Part model, mm, in its own coordinate system. A direction names the side the tool comes from. Coordinates: 2 decimals unless noted, no trailing zeros. Order: outer loops, then holes, each group sorted by start corner. A loop starts at its lowest first (then second) coordinate and runs counter-clockwise, first axis right, second up.
from build123d import *

# Parameters (mm, degrees)
FILLET_1_R = 1


with BuildPart() as part:
    # Эскиз1 → Повернуть1 (revolve)
    with BuildSketch(Plane.XY):
        Polygon((2.5, 0), (2.5, -30), (4.5, -30), (4.5, -0.828427125), (25.328427125, 20), (22.5, 20), align=None)
    revolve(axis=Axis((0, 0, 0), (0, 1, 0)))

    # Скругление1
    fillet_1_edges = [part.edges().sort_by_distance(p)[0] for p in [
        (-4.5, -30, 0),
        (-4.5, -0.828427125, 0),
        (-25.328427125, 20, 0),
    ]]
    fillet(fillet_1_edges, radius=FILLET_1_R)


solid = part.part
Q1. Which spindle directions (+Z, -Z, +X, -X, +Y, -Y) get a long thin tool onto all of the face, cutting with end or side? Do faces 1 (the face through (-0.54, -15.21, 2.44)), 2 (the face through (4.16, -14.93, 1.72)). Say none if no direction does.
Results list:
face 1: +Y, -Y
face 2: -Y
Q2. Cut at A-A on y = -16. Write the cut outline in (x, z).
Results list:
outline: circle Ø9 at (0, 0); hole circle Ø5 at (0, 0)
Q3. Cut at B-B on y = 4. Write the cut outline in (x, z), and give its area (3 significant figures).
Results list:
outline: circle Ø18.66 at (0, 0); hole circle Ø13 at (0, 0)
area: 141 mm2
Q4. Wall check: line 1 along X through (y, z) = (-18.75, 0); line 2 along X through (y, z) = (14.5, 13.5). Give the ranges that are in metal, low to high.
Results list:
line 1: x = -4.5 to -2.5, 2.5 to 4.5
line 2: x = -14.52 to -10.33, 10.33 to 14.52
Q5. Pin check, flat tips, straight feed: pin 1 Ø1 at (x, z) = (6.5, 18) entering from +Y; pin 2 Ø6 at (x, z) = (0, 0) entering from +Y; pin 3 Ø6 at (x, z) = (-7.5, 4) entering from +Y. Stop position of each tip, or through.
Results list:
pin 1: stops at y = 17.14
pin 2: stops at y = 0.5
pin 3: stops at y = 9
Q6. Mould opens along Z. For faces 3 (the face through (7.448, 2.734, 3.088)), 4 (the face through (-2, -30, 2)), 5 (the face through (5.43, 3.193, -1.71)) say: pulls with the +Z half, pulls with the -Z half, needs draft (parallel to the pull), parting line crosses it, or undercut.
Results list:
face 3: parting line crosses it
face 4: needs draft
face 5: undercut
